```python
from build123d import *

# Parameters (mm, degrees)
SKETCH1_W           = 50
SKETCH1_H           = 60
SKETCH1_W_2         = 47
SKETCH1_H_2         = 57
BOSS_EXTRUDE6_DEPTH = 40
SKETCH7_W           = 50
SKETCH7_H           = 60
BOSS_EXTRUDE8_DEPTH = 1.5
SKETCH8_W           = 10
SKETCH8_H           = 2
BOSS_EXTRUDE9_DEPTH = 50
SKETCH9_R           = 1.55
CUT_EXTRUDE1_DEPTH  = 3
SKETCH11_R          = 8.25
CUT_EXTRUDE3_DEPTH  = 1.5
SKETCH12_W          = 80
SKETCH12_H          = 42.428758989
CUT_EXTRUDE4_DEPTH  = 2
SKETCH13_W          = 92.772924303
SKETCH13_H          = 57.399075468
CUT_EXTRUDE5_DEPTH  = 42


with BuildPart() as part:
    # Sketch1 → Boss-Extrude6 (new body)
    with BuildSketch(Plane(origin=(0, 0, 0), x_dir=(1, 0, 0), z_dir=(0, 1, 0))):
        Rectangle(SKETCH1_W, SKETCH1_H)
        Rectangle(SKETCH1_W_2, SKETCH1_H_2, mode=Mode.SUBTRACT)
    extrude(amount=BOSS_EXTRUDE6_DEPTH)

    # Sketch7 → Boss-Extrude8 (add)
    with BuildSketch(Plane.XZ):
        Rectangle(SKETCH7_W, SKETCH7_H)
    extrude(amount=BOSS_EXTRUDE8_DEPTH)

    # Sketch8 → Boss-Extrude9 (add)
    with BuildSketch(Plane(origin=(25, 0, 0), x_dir=(0, 0, -1), z_dir=(1, 0, 0))):
        with Locations((-35, 39)):
            Rectangle(SKETCH8_W, SKETCH8_H)
        with Locations((35, 39)):
            Rectangle(SKETCH8_W, SKETCH8_H)
    extrude(amount=-BOSS_EXTRUDE9_DEPTH)

    # Sketch9 → Cut-Extrude1 (cut)
    with BuildSketch(Plane(origin=(0, 40, 0), x_dir=(1, 0, 0), z_dir=(0, 1, 0))):
        with Locations((-20, 35)):
            Circle(SKETCH9_R)
        with Locations((20, 35)):
            Circle(SKETCH9_R)
        with Locations((20, -35)):
            Circle(SKETCH9_R)
        with Locations((-20, -35)):
            Circle(SKETCH9_R)
    extrude(amount=-CUT_EXTRUDE1_DEPTH, mode=Mode.SUBTRACT)

    # Sketch11 → Cut-Extrude3 (cut)
    with BuildSketch(Plane.ZY.offset(25)):
        with Locations((0, 18.25)):
            Circle(SKETCH11_R)
    extrude(amount=-CUT_EXTRUDE3_DEPTH, mode=Mode.SUBTRACT)

    # Sketch12 → Cut-Extrude4 (cut)
    with BuildSketch(Plane.ZY.offset(25)):
        with Locations((0, 18.785620505)):
            Rectangle(SKETCH12_W, SKETCH12_H)
    extrude(amount=-CUT_EXTRUDE4_DEPTH, mode=Mode.SUBTRACT)

    # Sketch13 → Cut-Extrude5 (cut)
    with BuildSketch(Plane(origin=(25, 0, 0), x_dir=(0, 0, -1), z_dir=(1, 0, 0))):
        with Locations((0.049381319, 17.016100398)):
            Rectangle(SKETCH13_W, SKETCH13_H)
    extrude(amount=-CUT_EXTRUDE5_DEPTH, mode=Mode.SUBTRACT)


solid = part.part
```
For this review, take the finished solid that the model builds, in its own axes (mm). A direction names the side the tool comes from. Coordinates: 2 decimals unless noted, no trailing zeros. Order: outer loops, then holes, each group sorted by start corner. A loop starts at its lowest first (then second) coordinate and runs counter-clockwise, first axis right, second up. Notation, with made-up numbers: (-17.75, -13) - (22.25, -13) arc R15 cw to (22.25, 7) - close; hole circle Ø4 at (-10.75, 32.25). An arc over 180 degrees is marked (long way). Answer as a JSON object with one key per item and string values. Group by question number.
1. We need section A-A on y = 31. State the section outline as (x, z) points.
2. For faces 1 (the flat face through (-20, 40, -33)), 2 (the flat face through (-18.6, 38, -36)), 3 (the flat face through (-20, 19, 30)), 4 (the flat face through (-20, 39, 40)), 5 (the flat face through (-20, 0, 0)), list the 3-axis set-ups (+Z, -Z, +X, -X, +Y, -Y) from which the entire face can be reached by the end or side of a thin tool; tool diameter is ignored.
3. We need section B-B on x = -20. State the section outline as (y, z) points, then the cut area to 3 significant figures.
4. For probe 1 along Z at (x, y) = (-20, 38.7); probe 2 along X at (y, z) = (39.35, 35); probe 3 along Z at (x, y) = (-19.85, 36.5), list the stretches that pass through material, from the lowest coordinate up.
5. The part is to be moulded in two halves that separate along Z. For faces 6 (the flat face through (-23, -1, 0)), 7 (the cylindrical face through (-18.568, 39.014, -34.406)), 8 (the flat face through (-20, 19, -30)), say which applies: pulls with the +Z half, pulls with the -Z half, needs draft (parallel to the pull), parting line crosses it, or undercut.
6. We need section D-D on z = -3. State the section outline as (x, y) points, then the cut area to 3 significant figures.
7. We need section C-C on z = 35. State the section outline as (x, y) points, then the cut area to 3 significant figures.
8. Clearance check with flat-ended pins moving along their axes: P1, Ø1.8, axis at x = -20.5, y = 17, coming from the +Z side; P2, Ø1.8, axis at x = -19.5, z = 36, coming from the -Y side; P3, Ø3, axis at x = -19.5, z = -4, coming from the +Y side; P4, Ø1.9, axis at x = -20, z = 35, coming from the -Y side. State where each tip first meets the part, or that it passes through.
Final values:
{
 "1": {"outline": "(-23, -30) - (-17, -30) - (-17, -28.5) - (-23, -28.5) - close; (-23, 28.5) - (-17, 28.5) - (-17, 30) - (-23, 30) - close"},
 "2": {"face 1": "+Z, -Z, +X, -X, +Y", "face 2": "-Z, +X, -X, -Y", "face 3": "+Z, +X, -X, -Y", "face 4": "+Z, +X, -X, +Y, -Y", "face 5": "+X, -X, +Y"},
 "3": {"outline": "(-1.5, -30) - (38, -30) - (38, -33.45) - (40, -33.45) - (40, -28.5) - (0, -28.5) - (0, 28.5) - (40, 28.5) - (40, 33.45) - (38, 33.45) - (38, 30) - (-1.5, 30) - close; (38, -40) - (40, -40) - (40, -36.55) - (38, -36.55) - close; (38, 36.55) - (40, 36.55) - (40, 40) - (38, 40) - close", "area": "238 mm²"},
 "4": {"probe 1": "-40 to -36.55, -33.45 to -28.5, 28.5 to 33.45, 36.55 to 40", "probe 2": "-23 to -21.55, -18.45 to -17", "probe 3": "-30 to -28.5, 28.5 to 30"},
 "5": {"face 6": "needs draft", "face 7": "undercut", "face 8": "pulls with the -Z half"},
 "6": {"outline": "(-23, -1.5) - (-17, -1.5) - (-17, 0) - (-23, 0) - close", "area": "9.00 mm²"},
 "7": {"outline": "(-23, 38) - (-21.55, 38) - (-21.55, 40) - (-23, 40) - close; (-18.45, 38) - (-17, 38) - (-17, 40) - (-18.45, 40) - close", "area": "5.80 mm²"},
 "8": {"P1": "z = 30", "P2": "y = 38", "P3": "y = 0", "P4": "through"}
}
